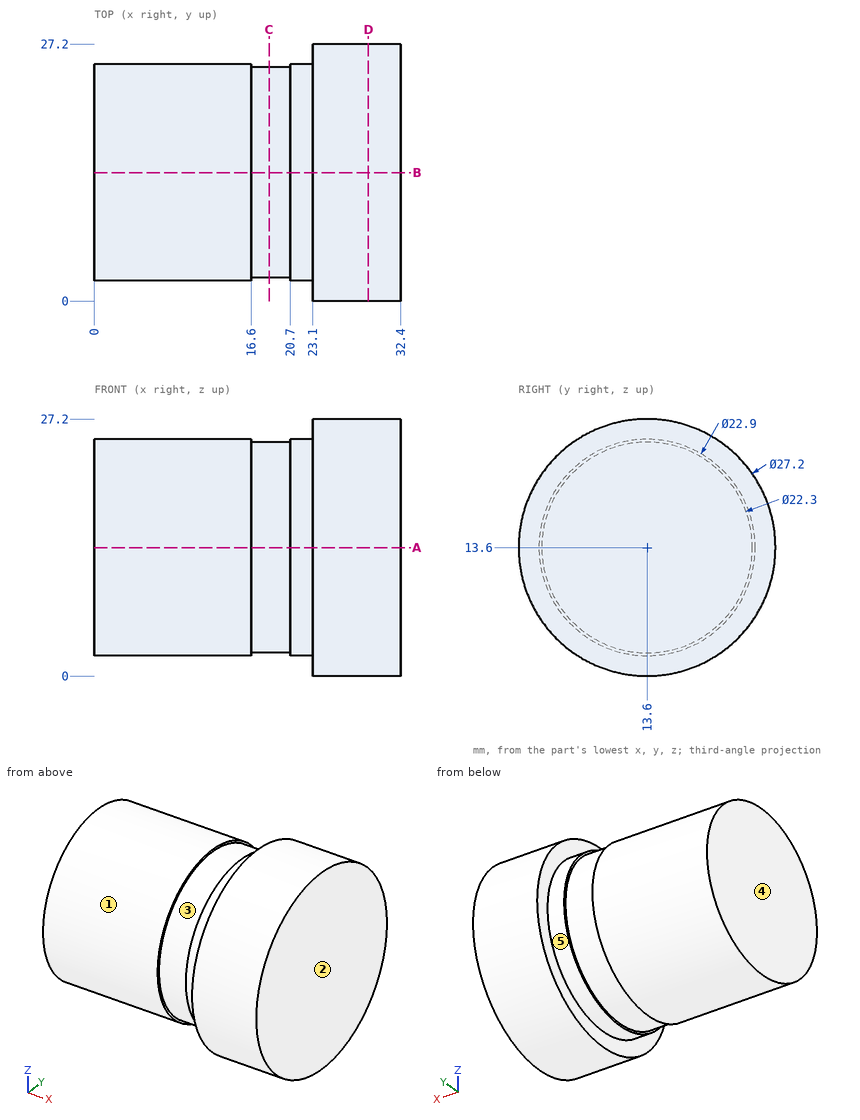
Here's the drawing with two shaded views (mm, measured from the low corner). I have some questions. A direction names the side the tool comes from. Coordinates: 2 decimals unless noted, no trailing zeros. Write each loop counter-clockwise with the first axis right and the second up, starting at its lowest first coordinate (ties: lowest second). Pieces come first, ordered by that corner, then holes. Notation, with made-up numbers: M 31,14.25 L 64,14.25 A18 cw 64,35.25 Z; hole C -35.75,-24.75 d6. An arc over 180 degrees is marked long. Answer as CSV lines item,"result".
Item 1: Imagine slicing it at D-D on x = 29. List the corners of the cut face in (y, z) for me.
Geometry results:
outline,"C 13.6,13.6 d27.2"
Item 2: Please list where these lines run through material, in increasing order: line 1 along X through (y, z) = (10.75, 25.25); line 2 along Y through (x, z) = (13, 11); line 3 along Z through (x, y) = (21, 14).
Geometry results:
line 1,"x = 23.1 to 32.4"
line 2,"y = 2.45 to 24.75"
line 3,"z = 2.16 to 25.04"
Item 3: On a 3-axis mill with a long thin cutter (end or side, diameter ignored), from which of +Z, -Z, +X, -X, +Y, -Y can I reach the whole of each face in a straight line? I mean the marked faces 1 and 2. Say none if no direction works.
Geometry results:
face 1,"-X"
face 2,"+Z, -Z, +X, +Y, -Y"
Item 4: Imagine slicing it at A-A on z = 13.6. List the corners of the cut face in (x, y) for me.
Geometry results:
outline,"M 0,2.15 L 16.6,2.15 L 16.6,2.45 L 20.7,2.45 L 20.7,2.15 L 23.1,2.15 L 23.1,0 L 32.4,0 L 32.4,27.2 L 23.1,27.2 L 23.1,25.05 L 20.7,25.05 L 20.7,24.75 L 16.6,24.75 L 16.6,25.05 L 0,25.05 Z"
Item 5: Imagine slicing it at C-C on x = 18.5. List the corners of the cut face in (y, z) for me, plus the area to 3 significant figures.
Geometry results:
outline,"C 13.6,13.6 d22.3"
area,"391 mm2"
Item 6: We'd pull the mould along X, two halves only. Please class the marked faces 3, 4 and 5: +X half, -X half, draft (parallel to the pull), parting line (faces both ways), or undercut.
Geometry results:
face 3,"undercut"
face 4,"-X half"
face 5,"draft"
Item 7: I'm going to push flat-ended pins straight in: P1, Ø5, axis at y = 20, z = 5, coming from the -X side; P2, Ø4, axis at x = 20.5, z = 19, coming from the -Y side; P3, Ø6, axis at x = 4, y = 12.5, coming from the +Z side; P4, Ø8, axis at x = 25.5, z = 4.5, coming from the -Y side. Where does each tip first touch, or does it pass through?
Geometry results:
P1,"stops at x = 0"
P2,"stops at y = 2.67"
P3,"stops at z = 25.05"
P4,"stops at y = 0.99"
